Geometry check sheet. Reference: the model listing, model coordinates, mm. Face numbers are marked on the shaded views. A direction names the side the tool comes from. Give positions to 0.01 mm unless a question says otherwise; leave off trailing zeros. Write each loop counter-clockwise with the first axis right and the second up, starting at its lowest first coordinate (ties: lowest second). Pieces come first, ordered by that corner, then holes. Notation, with made-up numbers: (81.25, -38.75) - (125.25, -38.75) arc R14 ccw to (125.25, -12.75) - close; hole circle Ø4 at (-13.75, -3.75). An arc over 180 degrees is marked (long way). One line per question, with ' | ' between items. Start each with the question number.
Q1. Section check C-C on z = 1.95. Record the boundary of the cut face in (x, y), and give its area (3 significant figures).
Q2. Thickness scan on L1, parallel to Y at x = 0, z = 3.7; L2, parallel to Y at x = 0, z = 0.9; L3, parallel to Y at x = 0.5, z = 3.6. Record the ranges inside material, lowest first. Write a range as [from, to].
Q3. Gauge pin test, flat ends, axial feed: P1, Ø1, axis at x = -1, z = 1.5, coming from the -Y side; P2, Ø4.5, axis at x = 2, y = 0, coming from the -Z side; P3, Ø1, axis at x = -1, z = 2.5, coming from the +Y side. Record the tip position at first contact, or that the pin passes through.
Q4. Set-up check for the marked faces 1 and 2: record each of +Z, -Z, +X, -X, +Y, -Y from which the full face is reachable in a straight line by a thin tool's end or side.
Q5. Release check for a two-part mould opening along X. For the marked faces 3 and 4 record: +X half, -X half, draft (parallel to the pull), parting line (faces both ways), or undercut.
```python
from build123d import *

# Parameters (mm, degrees)
SKIZZE1_R                       = 5
SKIZZE1_R_2                     = 2.5
AUFSATZ_LINEAR_AUSTRAGEN1_DEPTH = 4
VERRUNDUNG1_R                   = 0.2
SKIZZE2_R                       = 4.5
SKIZZE2_R_2                     = 3
SCHNITT_LINEAR_AUSTRAGEN1_DEPTH = 0.5
SCHNITT_LINEAR_START            = -0.5
SKIZZE3_R                       = 4.5
SKIZZE3_R_2                     = 3
SCHNITT_LINEAR_AUSTRAGEN2_DEPTH = 0.5


with BuildPart() as part:
    # Skizze1 → Aufsatz-Linear austragen1 (new body)
    with BuildSketch(Plane.XY):
        Circle(SKIZZE1_R)
        Circle(SKIZZE1_R_2, mode=Mode.SUBTRACT)
    extrude(amount=AUFSATZ_LINEAR_AUSTRAGEN1_DEPTH)

    # Verrundung1
    verrundung1_edges = [part.edges().sort_by_distance(p)[0] for p in [
        (-5, 0, 0),
        (-5, 0, 4),
        (-2.5, 0, 0),
        (-2.5, 0, 4),
    ]]
    fillet(verrundung1_edges, radius=VERRUNDUNG1_R)

    # Skizze2 → Schnitt-Linear austragen1 (cut)
    with BuildSketch(Plane(origin=(0, 0, 0), x_dir=(-1, 0, 0), z_dir=(0, 0, -1))):
        Circle(SKIZZE2_R)
        Circle(SKIZZE2_R_2, mode=Mode.SUBTRACT)
    extrude(amount=-SCHNITT_LINEAR_AUSTRAGEN1_DEPTH, mode=Mode.SUBTRACT)

    # Skizze3 → Schnitt-Linear austragen2 (cut)
    with BuildSketch(Plane.XY.offset(4).offset(SCHNITT_LINEAR_START)):
        with Locations(Location((0, 0, 0), (0, 0, 180))):
            Circle(SKIZZE3_R)
        with Locations(Location((0, 0, 0), (0, 0, 180))):
            Circle(SKIZZE3_R_2, mode=Mode.SUBTRACT)
    extrude(amount=SCHNITT_LINEAR_AUSTRAGEN2_DEPTH, mode=Mode.SUBTRACT)


solid = part.part
```
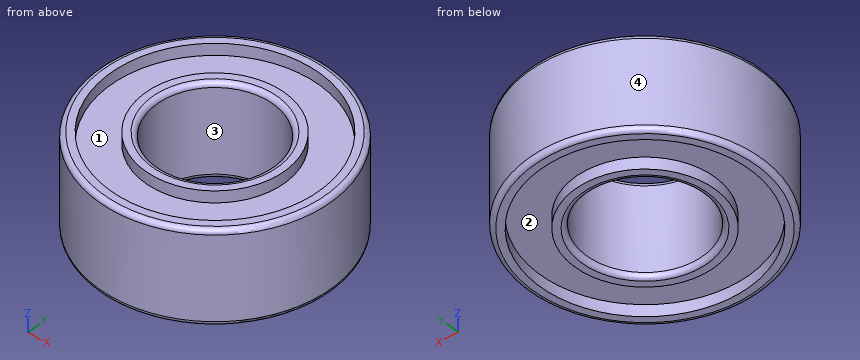
Working result:
1) outline: circle Ø10 at (0, 0); hole circle Ø5 at (0, 0) | area: 58.9 mm2
2) L1: y = [-5, -4.5], [-3, -2.5], [2.5, 3], [4.5, 5] | L2: y = [-5, -2.5], [2.5, 5] | L3: y = [-4.97, -4.47], [-2.96, -2.45], [2.45, 2.96], [4.47, 4.97]
3) P1: stops at y = -4.97 | P2: stops at z = 0 | P3: stops at y = 4.97
4) face 1: +Z | face 2: -Z
5) face 3: undercut | face 4: parting line
